CAD build for the part. Positions are in the model's coordinates, mm. A direction names the side the tool comes from. Give positions to 0.01 mm unless a question says otherwise; leave off trailing zeros. Loops run counter-clockwise (first coordinate to the right, second up) from the corner with the lowest first, then second, coordinate; pieces in that order, holes last.
Item 1: Probe probe 1 along X at (y, z) = (-2.5, 2.25); probe 2 along Z at (x, y) = (42, 4.75); probe 3 along X at (y, z) = (5, 7.25). List the from-to ranges inside material, lowest first.
Item 2: Saw through at B-B on y = 3.25. Give the cut face in (x, z), plus the area to 3 significant figures.
Item 3: Drop flat-ended pins along their axis: P1, Ø6, axis at x = 44, y = -2.5, coming from the +Z side; P2, Ø8, axis at x = 42.5, z = -5, coming from the -Y side; P3, Ø3, axis at y = -3.5, z = 5.5, coming from the -X side; P4, Ø0.5, axis at y = -5, z = -2, coming from the -X side. Give the stop position or say it passes through.
Item 4: Mould opens along X. For faces 1 (the flat face through (42, -4.5, 0)), 2 (the flat face through (25, 0, 9)), 3 (the cylindrical face through (-9, 0, 0)) say: released by +X, released by -X, zero draft, split by the parting line, or undercut.
Item 5: Which spindle directions (+Z, -Z, +X, -X, +Y, -Y) get a long thin tool onto all of the face, cutting with end or side? Do faces 4 (the flat face through (67.25, 0.08, -0.75)), 5 (the flat face through (49.2, -5.5, 0.6)), 6 (the flat face through (42, 4.5, 0)), 7 (the cylindrical face through (51.31, 0.08, 7.53)), 8 (the cylindrical face through (49.73, -4.99, -1.48)). Say none if no direction does.
Item 6: Saw through at A-A on x = 31.5. Give the cut face in (y, z).
from build123d import *

# Parameters (mm, degrees)
BOSS_EXTRUDE1_DEPTH = 5.5
SKETCH2_3_R         = 4.75
BOSS_EXTRUDE2_DEPTH = 4.5


with BuildPart() as part:
    # Sketch2 → Boss-Extrude1 (new, symmetric)
    with BuildSketch(Plane(origin=(0, 0, 0), x_dir=(1, 0, 0), z_dir=(0, 1, 0))):
        with BuildLine():
            Line((0, 9), (88, 9))
            ThreePointArc((88, 9), (90.828427125, 7.828427125), (92, 5))
            Line((92, 5), (92, -4.038605995))
            ThreePointArc((92, -4.038605995), (87.6201367, -9), (82.153827811, -5.269302997))
            ThreePointArc((82.153827811, -5.269302997), (80.773118265, -2.895756853), (78.347214076, -1.609261996))
            Line((78.347214076, -1.609261996), (55.847214076, 3.173260641))
            ThreePointArc((55.847214076, 3.173260641), (50.53042136, 0.871975682), (50.956106022, -4.905825787))
            ThreePointArc((50.956106022, -4.905825787), (51.292568558, -7.564087513), (49.030331222, -9))
            Line((49.030331222, -9), (0, -9))
            ThreePointArc((0, -9), (-9, 0), (0, 9))
        make_face()
        with BuildLine():
            Line((0, 8), (88, 8))
            ThreePointArc((88, 8), (90.121320344, 7.121320344), (91, 5))
            Line((91, 5), (91, -4.038605995))
            ThreePointArc((91, -4.038605995), (87.49610936, -8.007721199), (83.123062249, -5.023163597))
            ThreePointArc((83.123062249, -5.023163597), (81.466210794, -2.174908223), (78.555125766, -0.631114396))
            Line((78.555125766, -0.631114396), (56.055125766, 4.151408242))
            ThreePointArc((56.055125766, 4.151408242), (49.674974507, 1.389866291), (50.185796102, -5.543495472))
            ThreePointArc((50.185796102, -5.543495472), (50.387673623, -7.138452508), (49.030331222, -8))
            Line((49.030331222, -8), (0, -8))
            ThreePointArc((0, -8), (-8, 0), (0, 8))
        make_face(mode=Mode.SUBTRACT)
    extrude(amount=BOSS_EXTRUDE1_DEPTH, both=True)

    # Sketch2_3 → Boss-Extrude2 (add, symmetric)
    with BuildSketch(Plane(origin=(0, 0, 0), x_dir=(1, 0, 0), z_dir=(0, 1, 0))):
        with BuildLine():
            Line((0, 8), (88, 8))
            ThreePointArc((88, 8), (90.121320344, 7.121320344), (91, 5))
            Line((91, 5), (91, -4.038605995))
            ThreePointArc((91, -4.038605995), (87.49610936, -8.007721199), (83.123062249, -5.023163597))
            ThreePointArc((83.123062249, -5.023163597), (81.466210794, -2.174908223), (78.555125766, -0.631114396))
            Line((78.555125766, -0.631114396), (56.055125766, 4.151408242))
            ThreePointArc((56.055125766, 4.151408242), (49.674974507, 1.389866291), (50.185796102, -5.543495472))
            ThreePointArc((50.185796102, -5.543495472), (50.387673623, -7.138452508), (49.030331222, -8))
            Line((49.030331222, -8), (0, -8))
            ThreePointArc((0, -8), (-8, 0), (0, 8))
        make_face()
        with Locations(Location((0, 0, 0), (0, 0, 270))):
            Circle(SKETCH2_3_R, mode=Mode.SUBTRACT)
    extrude(amount=BOSS_EXTRUDE2_DEPTH, both=True)


solid = part.part
Results below:
1. probe 1: x = -8.71 to -4.18, 4.18 to 49.84, 79.94 to 92
1. probe 2: z = -9 to -8, 8 to 9
1. probe 3: x = -5.33 to -3.38, 50.33 to 51.42, 83.17 to 84.62, 89.38 to 90.83
2. outline: (0, -9) - (88, -9) arc R4 ccw to (92, -5) - (92, 4.04) arc R5 ccw to (82.15, 5.27) arc R5 cw to (78.35, 1.61) - (55.85, -3.17) arc R5 cw to (50.96, 4.91) arc R2.5 ccw to (49.03, 9) - (0, 9) arc R9 ccw to start; hole circle Ø9.5 at (0, 0)
2. area: 1,390 mm2
3. P1: stops at z = 9
3. P2: stops at y = -5.5
3. P3: stops at x = -8.06
3. P4: stops at x = -8.83
4. face 1: undercut
4. face 2: zero draft
4. face 3: released by -X
5. face 4: +Z, +Y, -Y
5. face 5: +Z, -Z, +X, -X, -Y
5. face 6: +Y
5. face 7: +Y, -Y
5. face 8: -Y
6. outline: (-5.5, -9) - (5.5, -9) - (5.5, -8) - (4.5, -8) - (4.5, 8) - (5.5, 8) - (5.5, 9) - (-5.5, 9) - (-5.5, 8) - (-4.5, 8) - (-4.5, -8) - (-5.5, -8) - close
